Can you work these out from the model? Positions are in its coordinate system, mm. A direction names the side the tool comes from. Coordinates: 2 decimals unless noted, no trailing zeros. Loops run counter-clockwise (first coordinate to the right, second up) from the corner with the lowest first, then second, coordinate; pieces in that order, holes last.
```python
from build123d import *

# Parameters (mm, degrees)
F2_R     = 13
F3_DEPTH = 280
F4_R     = 9
F5_DEPTH = 25
F7_DEPTH = 5


with BuildPart() as f1:
    # F0 (on Front) → F1 (revolve)
    with BuildSketch(Plane.XZ):
        Polygon((0, 41.006801), (0, 116.006801), (-15, 116.006801), (-15, 41.006801), (-20, 41.006801), (-20, 36.006801), (-15, 36.006801), (-15, -138.993199), (-20, -138.993199), (-20, -143.993199), (-15, -143.993199), (-15, -183.993199), (0, -183.993199), (0, -143.993199), (0, -138.993199), (0, 36.006801), align=None)
    revolve(axis=Axis((0, 0, -33.993199), (0, 0, -1)))

    # F2 (on face) → F3 (cut)
    with BuildSketch(Plane(origin=(0, 0, -183.993199), x_dir=(1, 0, 0), z_dir=(0, 0, -1))):
        Circle(F2_R)
    extrude(amount=-F3_DEPTH, mode=Mode.SUBTRACT)

    # F4 (on face) → F5 (cut)
    with BuildSketch(Plane.XY.offset(116.006801)):
        Circle(F4_R)
    extrude(amount=-F5_DEPTH, mode=Mode.SUBTRACT)

    # F6 (on Right) → F7 (join, symmetric)
    with BuildSketch(Plane.YZ):
        with BuildLine():
            ThreePointArc((11.778281, 0), (39.893063, -1.22572), (59.301081, 19.152508))
            ThreePointArc((59.301081, 19.152508), (31.186299, 20.378228), (11.778281, 0))
        make_face()
        with BuildLine():
            ThreePointArc((-11.181168, -111.06737), (-41.605309, -88.759159), (-79.289787, -86.980172))
            ThreePointArc((-79.289787, -86.980172), (-48.865646, -109.288382), (-11.181168, -111.06737))
        make_face()
    extrude(amount=F7_DEPTH, both=True)


solid = f1.part
```
(1) I want a section at D-D on y = -66. Write out the boundary of the cut face in (x, z).
Check values:
outline: (-5, -100.17) - (5, -100.17) - (5, -85.07) - (-5, -85.07) - close
(2) I'm going to push flat-ended pins straight in: pin 1 (10 mm diameter, centred on y = 16, z = 78.5, fed in from +X); pin 2 (0.9 mm diameter, centred on y = -12, z = -110.5, fed in from +X); pin 3 (1 mm diameter, centred on y = -14, z = -70, fed in from -X). Where does each tip first touch, or does it pass through?
Check values:
pin 1: stops at x = 10.2
pin 2: stops at x = 9.57
pin 3: stops at x = -6.54
(3) I want a section at A-A on y = 0. Write out the boundary of the cut face in (x, z).
Check values:
outline: (-20, -143.99) - (-15, -143.99) - (-15, -183.99) - (-13, -183.99) - (-13, 96.01) - (-9, 96.01) - (-9, 116.01) - (-15, 116.01) - (-15, 41.01) - (-20, 41.01) - (-20, 36.01) - (-15, 36.01) - (-15, -138.99) - (-20, -138.99) - close; (9, 96.01) - (13, 96.01) - (13, -183.99) - (15, -183.99) - (15, -143.99) - (20, -143.99) - (20, -138.99) - (15, -138.99) - (15, 36.01) - (20, 36.01) - (20, 41.01) - (15, 41.01) - (15, 116.01) - (9, 116.01) - close
(4) I want a section at B-B on z = 31. Write out the boundary of the cut face in (x, y).
Check values:
outline: circle Ø30 at (0, 0); hole circle Ø26 at (0, 0)
(5) I want a section at C-C on y = 47.5. Write out the boundary of the cut face in (x, z), then the cut area to 3 significant figures.
Check values:
outline: (-5, 3.05) - (5, 3.05) - (5, 22.65) - (-5, 22.65) - close
area: 196 mm2
(6) If I drill on probe 1 along X at (y, z) = (-1, -126); probe 2 along Y at (x, z) = (-5, -64); probe 3 along Y at (x, z) = (0, 106.5), over which ranges is the centre line in solid material (lowest first)?
Check values:
probe 1: x = -14.97 to -12.96, 12.96 to 14.97
probe 2: y = -14.14 to -12, 12 to 14.14
probe 3: y = -15 to -9, 9 to 15
(7) If we mould it in two halves opening along Z, with no side actions, what happens to faces 1 (the cylindrical face through (14.985, 0.66, -164.273)), 2 (the cylindrical face through (-14.307, 4.506, -52.718)), 3 (the flat face through (3, 15, 41.007))? For each: released by +Z, released by -Z, zero draft, split by the parting line, or undercut.
Check values:
face 1: zero draft
face 2: undercut
face 3: released by +Z
(8) Which directions (+Z, -Z, +X, -X, +Y, -Y) give clear straight access to the entire face, cutting with the end or side of a thin tool? Please do faces 4 (the flat face through (3, 15, -138.993)), 5 (the flat face through (6.5, -6.5, 116.007)), 6 (the cylindrical face through (4.336, -19.524, -141.528)), 7 (the cylindrical face through (4.336, -19.524, 38.472)).
Check values:
face 4: none
face 5: +Z, +X, -X, +Y, -Y
face 6: -Z
face 7: +Z
